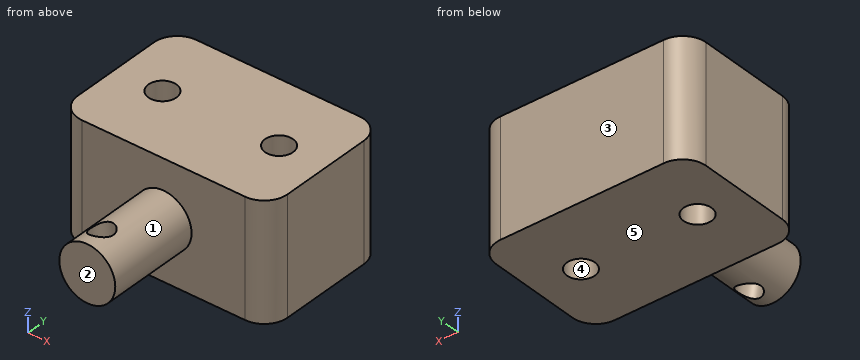
```python
from build123d import *

# Parameters (mm, degrees)
SKETCH_1_W               = 45
SKETCH_1_H               = 30
SKETCH_1_R               = 3
EXTRUDE_1_DEPTH          = 25
FILLET_1_R               = 5
SKETCH_2_R               = 6
EXTRUDE_2_DEPTH          = 20
SKETCH_3_R               = 2.5
CUT_EXTRUDE_1_DEPTH      = 17.21718091
CUT_EXTRUDE_1_DEPTH_BACK = 17.21718091


with BuildPart() as part:
    # Sketch 1 → Extrude 1 (new body)
    with BuildSketch(Plane.XY):
        Rectangle(SKETCH_1_W, SKETCH_1_H)
        with Locations((-12.5, 0)):
            Circle(SKETCH_1_R, mode=Mode.SUBTRACT)
        with Locations((12.5, 0)):
            Circle(SKETCH_1_R, mode=Mode.SUBTRACT)
    extrude(amount=EXTRUDE_1_DEPTH)

    # Fillet 1
    fillet_1_edges = [part.edges().sort_by_distance(p)[0] for p in [
        (22.5, -15, 12.5),
        (-22.5, -15, 12.5),
        (-22.5, 15, 12.5),
        (22.5, 15, 12.5),
    ]]
    fillet(fillet_1_edges, radius=FILLET_1_R)

    # Sketch 2 → Extrude 2 (add)
    with BuildSketch(Plane.XZ.offset(15)):
        with Locations((0, 12.5)):
            Circle(SKETCH_2_R)
    extrude(amount=EXTRUDE_2_DEPTH)

    # Sketch 3 → Cut-Extrude 1 (cut, two sides)
    with BuildSketch(Plane(origin=(-2.137625896, 0, 12.12307888), x_dir=(-0.984807753, 0, -0.173648178), z_dir=(0.173648178, 0, -0.984807753))) as cut_extrude_1_sk:
        with Locations((-2.170602221, -30)):
            Circle(SKETCH_3_R)
    extrude(amount=CUT_EXTRUDE_1_DEPTH, mode=Mode.SUBTRACT)
    extrude(cut_extrude_1_sk.sketch, amount=-CUT_EXTRUDE_1_DEPTH_BACK, mode=Mode.SUBTRACT)


solid = part.part
```
Input: part model. Units: mm. Frame: model coordinates. Face numbers are marked on the shaded views. A direction names the side the tool comes from. Round coordinates to 2 decimals unless told otherwise and drop trailing zeros. Order: outer loops, then holes, each group sorted by start corner. A loop starts at its lowest first (then second) coordinate and runs counter-clockwise, first axis right, second up. Notation, with made-up numbers: (-12, 67.5) - (35, 67.5) arc R16 cw to (35, 86.5) - close; hole circle Ø9 at (-0.5, 81). An arc over 180 degrees is marked (long way). One line per question, with ' | ' between items. Start each with the question number.
1) Ray query, probe 1 along Y at (x, z) = (-12.5, 20.25); probe 2 along Y at (x, z) = (8.5, 12.5); probe 3 along X at (y, z) = (-28, 10.25). Return the intervals inside material, ascending.
2) Cut plane A-A, the plane x = 12.5. Return the cut outline in (y, z).
3) Cut plane C-C, the plane z = 3.5. Return the cut outline in (x, y), then the cut area to 3 significant figures.
4) Cut plane B-B, the plane y = 0. Return the cut outline in (x, z), then the cut area to 3 significant figures.
5) Contact query for flat-ended pins moving along their axis: P1, Ø3, axis at x = 4, y = -29, coming from the +Z side; P2, Ø10, axis at y = -28.5, z = 10, coming from the +X side; P3, Ø4, axis at x = -3.5, y = -25.5, coming from the +Z side. Output: stop coordinate, or through.
6) Set-up query: the marked faces 1 and 2. Return all of +Z, -Z, +X, -X, +Y, -Y with unobstructed straight access to the full face (end or side cutting, diameter ignored); none if empty.
7) Cut plane D-D, the plane x = -4. Return the cut outline in (y, z).
8) Pull-direction query (Y, two-part tool) for the marked faces 3, 4 and 5; classes: +Y half, -Y half, draft (parallel to the pull), parting line (faces both ways), or undercut.
Worked out:
1) probe 1: y = -15 to -3, 3 to 15 | probe 2: y = -15 to 15 | probe 3: x = -5.56 to -1.13, 1.92 to 5.56
2) outline: (-15, 0) - (-3, 0) - (-3, 25) - (-15, 25) - close; (3, 0) - (15, 0) - (15, 25) - (3, 25) - close
3) outline: (-22.5, -10) arc R5 ccw to (-17.5, -15) - (17.5, -15) arc R5 ccw to (22.5, -10) - (22.5, 10) arc R5 ccw to (17.5, 15) - (-17.5, 15) arc R5 ccw to (-22.5, 10) - close; hole circle Ø6 at (-12.5, 0); hole circle Ø6 at (12.5, 0) | area: 1,270 mm^2
4) outline: (-22.5, 0) - (-15.5, 0) - (-15.5, 25) - (-22.5, 25) - close; (-9.5, 0) - (9.5, 0) - (9.5, 25) - (-9.5, 25) - close; (15.5, 0) - (22.5, 0) - (22.5, 25) - (15.5, 25) - close | area: 825 mm^2
5) P1: stops at z = 17.95 | P2: stops at x = 6 | P3: stops at z = 18.31
6) face 1: -Y | face 2: +Z, -Z, +X, -X, -Y
7) outline: (-35, 8.03) - (-15, 8.03) - (-15, 0) - (15, 0) - (15, 25) - (-15, 25) - (-15, 16.97) - (-35, 16.97) - close
8) face 3: +Y half | face 4: undercut | face 5: draft
